from build123d import *

# Parameters (mm, degrees)
SKETCH1_R                 = 11
SKETCH1_R_2               = 8
BOSS_EXTRUDE1_DEPTH       = 4.8
SKETCH2_W                 = 44.821432693
SKETCH2_H                 = 40.097165435
SKETCH2_R                 = 11
BOSS_EXTRUDE2_DEPTH       = 8.2
SKETCH3_W                 = 24
SKETCH3_H                 = 15
SKETCH3_R                 = 8
BOSS_EXTRUDE3_DEPTH       = 5
BOSS_EXTRUDE4_OUTLINE_W   = 48.178567307
BOSS_EXTRUDE4_OUTLINE_H   = 40.5
BOSS_EXTRUDE4_OUTLINE_R   = 1.6
BOSS_EXTRUDE4_OUTLINE_R_2 = 6.35
BOSS_EXTRUDE4_OUTLINE_R_3 = 2.1
BOSS_EXTRUDE4_DEPTH       = 5
BOSS_EXTRUDE5_DEPTH       = 5
SKETCH6_W                 = 48.178567307
SKETCH6_H                 = 17.568704936
BOSS_EXTRUDE6_DEPTH       = 5
SKETCH8_R                 = 2
CUT_EXTRUDE1_DEPTH        = 127.437257167
CUT_EXTRUDE2_START        = -23.95
CUT_EXTRUDE2_OUTLINE_W    = 64.98154514
CUT_EXTRUDE2_OUTLINE_H    = 102.7
CUT_EXTRUDE2_OUTLINE_R    = 11
CUT_EXTRUDE2_DEPTH        = 23.95
CUT_EXTRUDE2_START_2      = -45.3
CUT_EXTRUDE2_2_DEPTH      = 21.35
SKETCH13_W                = 48.029963693
SKETCH13_H                = 72.7
CUT_EXTRUDE5_DEPTH        = 100
SKETCH14_W                = 52.01845486
SKETCH14_H                = 5
CUT_EXTRUDE6_DEPTH        = 100
SKETCH15_W                = 24
SKETCH15_H                = 10
BOSS_EXTRUDE7_DEPTH       = 10
SKETCH16_R                = 2
CUT_EXTRUDE7_DEPTH        = 30
SKETCH17_W                = 28.01845486
SKETCH17_H                = 5.3
CUT_EXTRUDE11_DEPTH       = 100
SKETCH18_W                = 24
SKETCH18_H                = 4.59
CUT_EXTRUDE12_DEPTH       = 43.450839953
SKETCH19_W                = 4.5
SKETCH19_H                = 7
BOSS_EXTRUDE8_DEPTH       = 24
SKETCH20_W                = 24
SKETCH20_H                = 7
BOSS_EXTRUDE9_DEPTH       = 15.3
SKETCH21_R                = 2
CUT_EXTRUDE13_DEPTH       = 39
SKETCH22_W                = 24
SKETCH22_H                = 5.41
CUT_EXTRUDE14_DEPTH       = 39
BOSS_EXTRUDE11_START      = -7
BOSS_EXTRUDE11_DEPTH      = 7
SKETCH26_W                = 4.5
SKETCH26_H                = 25
BOSS_EXTRUDE12_DEPTH      = 14.5
BOSS_EXTRUDE13_START      = -4.5
SKETCH27_R                = 8
BOSS_EXTRUDE13_DEPTH      = 4.5
SKETCH28_R                = 8
CUT_EXTRUDE15_DEPTH       = 4.5


# Read off the part's stored shape, not the designer's step: Boss-Extrude4, Cut-Extrude2
with BuildPart() as part:
    # Sketch1 → Boss-Extrude1 (new body)
    # profile 1 of 2: a face of its own
    with BuildSketch(Plane.XY):
        Polygon((0, 0), (93, 0), (93, 102.7), (0, 102.7), (0, 30), (-24, 30), (-24, 15), (0, 15), align=None)
        with Locations((15, 10.5)):
            Circle(SKETCH1_R, mode=Mode.SUBTRACT)
        with Locations((70, 72)):
            Circle(SKETCH1_R, mode=Mode.SUBTRACT)
    # profile 2 of 2: a face of its own
    with BuildSketch(Plane.XY):
        with BuildLine():
            ThreePointArc((26, 10.5), (8.48332569, 19.36188219), (11.721280738, 0))
            Line((11.721280738, 0), (18.278719262, 0))
            ThreePointArc((18.278719262, 0), (23.86188219, 3.98332569), (26, 10.5))
        make_face()
        with Locations((15, 10.5)):
            Circle(SKETCH1_R_2, mode=Mode.SUBTRACT)
    extrude(amount=BOSS_EXTRUDE1_DEPTH)

    # Sketch2 → Boss-Extrude2 (add)
    with BuildSketch(Plane.XY.offset(4.8)):
        with Locations((70.589283654, 72.714594712)):
            Rectangle(SKETCH2_W, SKETCH2_H)
        with Locations((70, 72)):
            Circle(SKETCH2_R, mode=Mode.SUBTRACT)
    extrude(amount=BOSS_EXTRUDE2_DEPTH)

    # Sketch3 → Boss-Extrude3 (add)
    # profile 1 of 2: a face of its own
    with BuildSketch(Plane.XY.offset(4.8)):
        with Locations((-12, 22.5)):
            Rectangle(SKETCH3_W, SKETCH3_H)
    # profile 2 of 2: a face of its own
    with BuildSketch(Plane.XY.offset(4.8)):
        Polygon((0, 30), (0, 15), (0, 0), (93, 0), (93, 52.666011994), (48.178567307, 52.666011994), (0, 52.666011994), align=None)
        with Locations((15, 10.5)):
            Circle(SKETCH3_R, mode=Mode.SUBTRACT)
    extrude(amount=BOSS_EXTRUDE3_DEPTH)

    # Boss-Extrude4 outline → Boss-Extrude4 (add)
    # profile 1 of 2: a face of its own
    with BuildSketch(Plane.XZ.offset(-75.23471693)):
        with Locations((24.089283654, 25.05)):
            Rectangle(BOSS_EXTRUDE4_OUTLINE_W, BOSS_EXTRUDE4_OUTLINE_H)
        with Locations((22.860422048, 23.3)):
            Circle(BOSS_EXTRUDE4_OUTLINE_R, mode=Mode.SUBTRACT)
        with Locations((38.360422048, 30.3)):
            Circle(BOSS_EXTRUDE4_OUTLINE_R_2, mode=Mode.SUBTRACT)
        with Locations((30.610422048, 36.723393759)):
            Circle(BOSS_EXTRUDE4_OUTLINE_R, mode=Mode.SUBTRACT)
        with Locations((46.110422048, 36.723393759)):
            Circle(BOSS_EXTRUDE4_OUTLINE_R, mode=Mode.SUBTRACT)
    # profile 2 of 2: a face of its own
    with BuildSketch(Plane.XZ.offset(-75.23471693)):
        with Locations((51.783815806, 31.05)):
            Circle(BOSS_EXTRUDE4_OUTLINE_R_3)
    extrude(amount=BOSS_EXTRUDE4_DEPTH)

    # Sketch5 → Boss-Extrude5 (add)
    with BuildSketch(Plane(origin=(48.178567307, 0, 0), x_dir=(0, 0, -1), z_dir=(1, 0, 0))):
        Polygon((-45.3, 75.23471693), (-13, 92.763177429), (-4.8, 92.763177429), (-4.8, 70.23471693), (-45.3, 70.23471693), align=None)
    extrude(amount=-BOSS_EXTRUDE5_DEPTH)

    # Sketch6 → Boss-Extrude6 (add)
    with BuildSketch(Plane.XY.offset(4.8)):
        with Locations((24.089283654, 61.450364462)):
            Rectangle(SKETCH6_W, SKETCH6_H)
    extrude(amount=BOSS_EXTRUDE6_DEPTH)

    # Sketch8 → Cut-Extrude1 (cut, through all)
    with BuildSketch(Plane(origin=(0, 30, 0), x_dir=(1, 0, 0), z_dir=(0, 1, 0))):
        with Locations(Location((-12, -4.9, 0), (0, 0, 180))):
            Circle(SKETCH8_R)
    extrude(amount=-CUT_EXTRUDE1_DEPTH, mode=Mode.SUBTRACT)

    # Cut-Extrude2 outline → Cut-Extrude2 (cut)
    with BuildSketch(Plane(origin=(0, 0, 0), x_dir=(-1, 0, 0), z_dir=(0, 0, -1)).offset(CUT_EXTRUDE2_START)):
        with Locations((-60.50922743, 51.35)):
            Rectangle(CUT_EXTRUDE2_OUTLINE_W, CUT_EXTRUDE2_OUTLINE_H)
        with Locations((-70, 72)):
            Circle(CUT_EXTRUDE2_OUTLINE_R, mode=Mode.SUBTRACT)
    extrude(amount=CUT_EXTRUDE2_DEPTH, mode=Mode.SUBTRACT)

    # Cut-Extrude2 2 outline → Cut-Extrude2 2 (cut)
    with BuildSketch(Plane(origin=(0, 0, 0), x_dir=(-1, 0, 0), z_dir=(0, 0, -1)).offset(CUT_EXTRUDE2_START_2)):
        Polygon((-28.01845486, 70.23471693), (-28.01845486, 75.23471693), (-43.178567307, 75.23471693), (-43.178567307, 92.763177429), (-48.178567307, 92.763177429), (-48.178567307, 70.23471693), align=None)
    extrude(amount=CUT_EXTRUDE2_2_DEPTH, mode=Mode.SUBTRACT)

    # Sketch13 → Cut-Extrude5 (cut)
    with BuildSketch(Plane.ZY):
        with Locations((24.014981847, 66.35)):
            Rectangle(SKETCH13_W, SKETCH13_H)
    extrude(amount=-CUT_EXTRUDE5_DEPTH, mode=Mode.SUBTRACT)

    # Sketch14 → Cut-Extrude6 (cut)
    with BuildSketch(Plane.XY.offset(9.8)):
        with Locations((2.00922743, 27.5)):
            Rectangle(SKETCH14_W, SKETCH14_H)
    extrude(amount=-CUT_EXTRUDE6_DEPTH, mode=Mode.SUBTRACT)

    # Sketch15 → Boss-Extrude7 (add)
    with BuildSketch(Plane.XY.offset(9.8)):
        with Locations((-12, 20)):
            Rectangle(SKETCH15_W, SKETCH15_H)
    extrude(amount=BOSS_EXTRUDE7_DEPTH)

    # Sketch16 → Cut-Extrude7 (cut)
    with BuildSketch(Plane(origin=(0, 25, 0), x_dir=(1, 0, 0), z_dir=(0, 1, 0))):
        with Locations(Location((-12, -14.8, 0), (0, 0, 270))):
            Circle(SKETCH16_R)
    extrude(amount=-CUT_EXTRUDE7_DEPTH, mode=Mode.SUBTRACT)

    # Sketch17 → Cut-Extrude11 (cut)
    with BuildSketch(Plane(origin=(0, 25, 0), x_dir=(1, 0, 0), z_dir=(0, 1, 0))):
        with Locations((14.00922743, -7.15)):
            Rectangle(SKETCH17_W, SKETCH17_H)
    extrude(amount=-CUT_EXTRUDE11_DEPTH, mode=Mode.SUBTRACT)

    # Sketch18 → Cut-Extrude12 (cut, through all)
    with BuildSketch(Plane(origin=(0, 0, 0), x_dir=(-1, 0, 0), z_dir=(0, 0, -1))):
        with Locations((12, 17.295)):
            Rectangle(SKETCH18_W, SKETCH18_H)
    extrude(amount=-CUT_EXTRUDE12_DEPTH, mode=Mode.SUBTRACT)

    # Sketch19 → Boss-Extrude8 (add)
    with BuildSketch(Plane.ZY):
        with Locations((2.25, 8.59)):
            Rectangle(SKETCH19_W, SKETCH19_H)
    extrude(amount=BOSS_EXTRUDE8_DEPTH)

    # Sketch20 → Boss-Extrude9 (add)
    with BuildSketch(Plane.XY.offset(4.5)):
        with Locations((-12, 8.59)):
            Rectangle(SKETCH20_W, SKETCH20_H)
    extrude(amount=BOSS_EXTRUDE9_DEPTH)

    # Sketch21 → Cut-Extrude13 (cut)
    with BuildSketch(Plane(origin=(0, 25, 0), x_dir=(1, 0, 0), z_dir=(0, 1, 0))):
        with Locations(Location((-12, -4.9, 0), (0, 0, 180))):
            Circle(SKETCH21_R)
        with Locations(Location((-12, -14.8, 0), (0, 0, 270))):
            Circle(SKETCH21_R)
    extrude(amount=-CUT_EXTRUDE13_DEPTH, mode=Mode.SUBTRACT)

    # Sketch22 → Cut-Extrude14 (cut)
    with BuildSketch(Plane(origin=(0, 0, 0), x_dir=(-1, 0, 0), z_dir=(0, 0, -1))):
        with Locations((12, 22.295)):
            Rectangle(SKETCH22_W, SKETCH22_H)
    extrude(amount=-CUT_EXTRUDE14_DEPTH, mode=Mode.SUBTRACT)

    # Sketch25 → Boss-Extrude11 (add)
    with BuildSketch(Plane.XZ.offset(-5.09).offset(BOSS_EXTRUDE11_START)):
        Polygon((0, 4.5), (0, 12.15), (5.681243584, 4.5), align=None)
    extrude(amount=BOSS_EXTRUDE11_DEPTH)

    # Sketch26 → Boss-Extrude12 (add)
    with BuildSketch(Plane(origin=(28.01845486, 0, 0), x_dir=(0, 0, -1), z_dir=(1, 0, 0))):
        with Locations((-2.25, 12.5)):
            Rectangle(SKETCH26_W, SKETCH26_H)
    extrude(amount=BOSS_EXTRUDE12_DEPTH)

    # Sketch27 → Boss-Extrude13 (add)
    with BuildSketch(Plane.XY.offset(4.5).offset(BOSS_EXTRUDE13_START)):
        with Locations((15, 10.5)):
            Circle(SKETCH27_R)
    extrude(amount=BOSS_EXTRUDE13_DEPTH)

    # Sketch28 → Cut-Extrude15 (cut)
    with BuildSketch(Plane.XY.offset(4.5)):
        with Locations((29.49845486, 10.5)):
            Circle(SKETCH28_R)
    extrude(amount=-CUT_EXTRUDE15_DEPTH, mode=Mode.SUBTRACT)


solid = part.part
Verification items for the finished model (mm, model axes). A direction names the side the tool comes from. Round coordinates to 2 decimals unless told otherwise and drop trailing zeros. Order: outer loops, then holes, each group sorted by start corner. A loop starts at its lowest first (then second) coordinate and runs counter-clockwise, first axis right, second up.
1. Section check C-C on y = 10.5. Record the cut outline in (x, z).
Final values:
outline: (-24, 0) - (21.5, 0) - (21.5, 4.5) - (5.68, 4.5) - (0, 12.15) - (0, 19.8) - (-24, 19.8) - close; (37.5, 0) - (42.52, 0) - (42.52, 4.5) - (37.5, 4.5) - close; hole circle Ø4 at (-12, 4.9); hole circle Ø4 at (-12, 14.8)
2. Section check B-B on x = -12. Record the cut outline in (y, z), then the cut area to 3 significant figures.
Final values:
outline: (5.09, 0) - (12.09, 0) - (12.09, 2.9) - (5.09, 2.9) - close; (5.09, 6.9) - (12.09, 6.9) - (12.09, 12.8) - (5.09, 12.8) - close; (5.09, 16.8) - (12.09, 16.8) - (12.09, 19.8) - (5.09, 19.8) - close
area: 82.6 mm2
3. Section check D-D on x = 29.5. Record the cut outline in (y, z), then the cut area to 3 significant figures.
Final values:
outline: (0, 0) - (2.5, 0) - (2.5, 4.5) - (0, 4.5) - close; (18.5, 0) - (25, 0) - (25, 4.5) - (18.5, 4.5) - close
area: 40.5 mm2
4. Section check A-A on z = 14.8. Record the cut outline in (x, y), then the cut area to 3 significant figures.
Final values:
outline: (-24, 5.09) - (-14, 5.09) - (-14, 12.09) - (-24, 12.09) - close; (-10, 5.09) - (0, 5.09) - (0, 12.09) - (-10, 12.09) - close
area: 140 mm2
5. Release check for a two-part mould opening along X. For faces 1 (the flat face through (-24, 9, 10)), 2 (the flat face through (0, 9, 16)), 3 (the cylindrical face through (-10.526, 8.639, 6.252)) record: +X half, -X half, draft (parallel to the pull), parting line (faces both ways), or undercut.
Final values:
face 1: -X half
face 2: +X half
face 3: undercut
6. Access from +Z, -Z, +X, -X, +Y, -Y to the whole of each face (thin tool, end or side, straight path). Record for faces 4 (the flat face through (0, 18, 2)), 5 (the flat face through (0, 3, 2)), 6 (the flat face through (21, 0, 2)).
Final values:
face 4: +Z, -Z, -X, +Y
face 5: +Z, -Z, -X, -Y
face 6: +Z, -Z, +X, -X, -Y
7. Thickness scan on L1, parallel to X at y = 7.5, z = 14.8; L2, parallel to Y at x = -12.5, z = 9.25; L3, parallel to Z at x = 6, y = 20.75. Record the ranges inside material, lowest first.
Final values:
L1: x = -24 to -14, -10 to 0
L2: y = 5.09 to 12.09
L3: z = 0 to 4.5
8. Go/stop test with flat-tipped pins: P1, Ø5, axis at y = 19, z = 3, coming from the -X side; P2, Ø5, axis at x = -9, y = 13, coming from the -Z side; P3, Ø2, axis at y = 10, z = 14.5, coming from the +X side; P4, Ø10, axis at x = -5, z = 9, coming from the -Y side. Record where each tip stops, or that it passes through.
Final values:
P1: stops at x = 0
P2: stops at z = 0
P3: stops at x = 0
P4: stops at y = 5.09
